Model file for the job. Use its own axes, mm. Give positions to 0.01 mm unless a question says otherwise; leave off trailing zeros. Answer as CSV lines item,"result". Start each with the question number.
Item 1: Pull direction X, two halves, no side cores. Call faces 1 (the flat face through (-14, 22, 0)), 2 (the cylindrical face through (-6.88, -30.99, 11.97)): pulls with the +X half, pulls with the -X half, needs draft (parallel to the pull), parting line crosses it, or undercut.
Item 2: Drill centre lines: L1, parallel to X at y = -0.5, z = 15; L2, parallel to X at y = -14.5, z = 16.75. Where is each one in solid material? Low to high. Write a range as from..to.
Item 3: Pin check, flat tips, straight feed: pin 1 (5 mm diameter, centred on x = -21, z = 4.5, fed in from +Y); pin 2 (5 mm diameter, centred on x = -10.5, z = 2, fed in from -Y); pin 3 (2 mm diameter, centred on y = -17.5, z = 9, fed in from +X). Stop position of each tip, or through.
from build123d import *

# Parameters (mm, degrees)
F0_R     = 31.742786
F1_DEPTH = 21.59
F2_R     = 5.08
F3_R     = 2.54


with BuildPart() as f1:
    # F0 (on Top) → F1 (new body)
    with BuildSketch(Plane.XY):
        Circle(F0_R)
        with BuildLine():
            ThreePointArc((18.484382, 17.87337), (23.837034, 9.63979), (25.712443, 0))
            ThreePointArc((25.712443, 0), (23.118518, -11.254504), (15.860104, -20.238252))
            ThreePointArc((15.860104, -20.238252), (8.389125, -24.305397), (0, -25.712443))
            ThreePointArc((0, -25.712443), (-9.855162, -23.748801), (-18.205059, -18.157797))
            ThreePointArc((-18.205059, -18.157797), (-23.76159, -9.824286), (-25.712443, 0))
            ThreePointArc((-25.712443, 0), (-23.263593, 10.951483), (-16.383499, 19.81693))
            ThreePointArc((-16.383499, 19.81693), (-8.705977, 24.193712), (0, 25.712443))
            ThreePointArc((0, 25.712443), (10.038967, 23.671689), (18.484382, 17.87337))
        make_face(mode=Mode.SUBTRACT)
    extrude(amount=F1_DEPTH)

    # F2
    f2_edges = [f1.edges().sort_by_distance(p)[0] for p in [
        (-31.742786, 0, 0),
    ]]
    fillet(f2_edges, radius=F2_R)

    # F3
    f3_edges = [f1.edges().sort_by_distance(p)[0] for p in [
        (-31.742786, 0, 21.59),
    ]]
    fillet(f3_edges, radius=F3_R)


solid = f1.part
Responses:
1,face 1,"needs draft"
1,face 2,"parting line crosses it"
2,L1,"-31.74..-25.71, 25.71..31.74"
2,L2,"-28.24..-21.23, 21.23..28.24"
3,pin 1,"y = 25.77"
3,pin 2,"y = -30.34"
3,pin 3,"x = 27.12"
